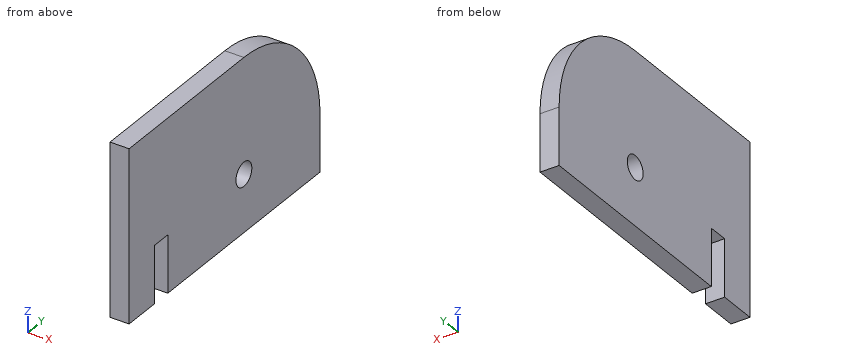
from build123d import *

# Parameters (mm, degrees)
SKETCH1_R           = 7.9375
BOSS_EXTRUDE1_DEPTH = 6.35


with BuildPart() as part:
    # Sketch1 → Boss-Extrude1 (new body, symmetric)
    with BuildSketch(Plane(origin=(0, 0, 0), x_dir=(0, 0, -1), z_dir=(1, 0, 0))):
        with BuildLine():
            Line((0, -76.2), (38.1, -76.2))
            Line((38.1, -76.2), (38.1, 76.2))
            Line((38.1, 76.2), (0, 76.2))
            ThreePointArc((0, 76.2), (-53.881536726, 53.881536726), (-76.2, 0))
            Line((-76.2, 0), (-76.2, -114.935))
            Line((-76.2, -114.935), (38.1, -114.935))
            Line((38.1, -114.935), (38.1, -89.535))
            Line((38.1, -89.535), (0, -89.535))
            Line((0, -89.535), (0, -76.2))
        make_face()
        Circle(SKETCH1_R, mode=Mode.SUBTRACT)
    extrude(amount=BOSS_EXTRUDE1_DEPTH, both=True)


solid = part.part
Geometry check sheet. Reference: the model listing, model coordinates, mm. Coordinates: 2 decimals unless noted, no trailing zeros. Write each loop counter-clockwise with the first axis right and the second up, starting at its lowest first coordinate (ties: lowest second). Pieces come first, ordered by that corner, then holes. Notation, with made-up numbers: (83.5, 89.5) -> (117.5, 89.5) arc R30 cw to (117.5, 119.5) -> close; hole circle Ø9 at (-22, 52.25). An arc over 180 degrees is marked (long way). One line per question, with ' | ' between items.
1. Cross-section at A-A on x = 0. Record the cut outline in (y, z) (1 decimal).
Answers:
outline: (-114.9, -38.1) -> (-89.5, -38.1) -> (-89.5, 0) -> (-76.2, 0) -> (-76.2, -38.1) -> (76.2, -38.1) -> (76.2, 0) arc R76.2 ccw to (0, 76.2) -> (-114.9, 76.2) -> close; hole circle Ø15.9 at (0, 0)
2. Depth check by flat-ended pin: pin 1 Ø1.5 at (x, z) = (2, 58) entering from +Y. Enter the tip coordinate at first touch or a pass-through.
Answers:
pin 1: stops at y = 50.29
3. Cross-section at C-C on z = 50. Record the cut outline in (x, y) (3 decimals).
Answers:
outline: (-6.35, -114.935) -> (6.35, -114.935) -> (6.35, 57.502) -> (-6.35, 57.502) -> close
4. Thickness scan on probe 1 along Y at (x, z) = (3.5, -20) (3 decimals); probe 2 along Y at (x, z) = (-4, -4.5) (3 decimals); probe 3 along Z at (x, y) = (-2.5, -78). Record the ranges inside material, lowest first. Write a range as from..to.
Answers:
probe 1: y = -114.935..-89.535, -76.2..76.2 | probe 2: y = -114.935..-89.535, -76.2..-6.539, 6.539..76.2 | probe 3: z = 0..76.2
5. Cross-section at B-B on y = 49.5. Record the cut outline in (x, z).
Answers:
outline: (-6.35, -38.1) -> (6.35, -38.1) -> (6.35, 57.93) -> (-6.35, 57.93) -> close
